Input: part model. Units: mm. Frame: model coordinates. A direction names the side the tool comes from. Round coordinates to 2 decimals unless told otherwise and drop trailing zeros. Loops run counter-clockwise (first coordinate to the right, second up) from the corner with the lowest first, then second, coordinate; pieces in that order, holes last. Notation, with made-up numbers: (-8.5, 54) -> (16.5, 54) arc R23 ccw to (16.5, 90) -> close; hole circle Ø8 at (-6, 47). An arc over 180 degrees is marked (long way). Answer as a JSON object with one key per item and string values.
Autodesk Fusion 360 part; units mm, degrees
sketch "Sketch1" plane through (0, 0, 0) normal (0, 0, 1) x (1, 0, 0)
  circle A0 centre (0, 0) radius 29.25
  circle A1 centre (0, 0) radius 31.25
  dimension "d1" = 58.5
  dimension "d2" = 2
ref_plane "WorkPlane1" through (0, 0, 10) normal (0, 0, 1) x (1, 0, 0)
sketch "Sketch2" plane through (0, 0, 10) normal (0, 0, 1) x (1, 0, 0)
  circle A0 centre (0, 0) radius 18.9
  circle A1 centre (0, 0) radius 20.9
  dimension "d4" = 37.8
  dimension "d5" = 2
sketch "Sketch3" plane through (0, 0, 0) normal (0, 1, 0) x (1, 0, 0)
  line L0 (-29.25, 0) -> (29.25, 0)
  line L1 (-31.25, 0) -> (31.25, 0)
  line L2 (-18.9, -10) -> (18.9, -10)
  line L3 (-20.9, -10) -> (20.9, -10)
  line L4 (-31.25, 0) -> (-20.9, -10)
  line L5 (-18.9, -10) -> (-29.25, 0)
  line L6 (0, 0) -> (0, -30) construction
revolve "Revolve1" add sketch "Sketch3" angle 360 about axis through (0, 0, 0) along (0, 0, 1)
extrude "Extrude1" add sketch "Sketch2" along normal blind 25
extrude "Extrude2" add sketch "Sketch1" against normal blind 25
fillet "Fillet1" radius 10 1 edges at (-27.2706, 10.5773, 0)
fillet "Fillet2" radius 10 2 edges at (-17.621, 6.8345, 10) (-19.4856, 7.5578, 10)
fillet "Fillet3" radius 10 1 edges at (-29.1352, 11.3005, 0)
1) Section A-A, the plane z = -13. Output: boundary loops of the cut face in (x, y).
Output:
{"outline": "circle Ø62.5 at (0, 0); hole circle Ø58.5 at (0, 0)"}
2) Ray query, probe 1 along X at (y, z) = (0, -11.75); probe 2 along X at (y, z) = (0, 24). Return the intervals inside material, ascending.
Output:
{"probe 1": "x = -31.25 to -29.25, 29.25 to 31.25", "probe 2": "x = -20.9 to -18.9, 18.9 to 20.9"}
3) Contact query for flat-ended pins moving along their axis: P1, Ø6, axis at x = 11, z = -9.5, coming from the -Y side; P2, Ø1.5, axis at y = -14, z = 1.5, coming from the +X side; P3, Ø8, axis at y = 23.5, z = -19, coming from the +X side. Output: stop coordinate, or through.
Output:
{"P1": "stops at y = -30.21", "P2": "stops at x = 26.57", "P3": "stops at x = 24.42"}
4) Reachability of faces 1 (the face through (-31.22, 1.37, -14.48)), 2 (the face through (-6.341, -28.554, -14.476)), 3 (the face through (-15.4, -14.13, 24.48)) from +Z, -Z, +X, -X, +Y, -Y: full face, straight path, thin tool, end or side. Return the list, or none.
Output:
{"face 1": "+Z, -Z", "face 2": "-Z", "face 3": "+Z"}
5) Draft query along X for faces 4 (the face through (21, -21, -25)), 5 (the face through (5.25, -23.641, 6.795)), 6 (the face through (4.816, -21.689, 6.795)). Return one class per face: +X half, -X half, draft (parallel to the pull), parting line (faces both ways), or undercut.
Output:
{"face 4": "draft", "face 5": "parting line", "face 6": "undercut"}
